from build123d import *

# Parameters (mm, degrees)
F1_DEPTH = 5
F2_R     = 0.7
F3_R     = 2
F4_SIZE  = 0.4
F5_R     = 1.5
F6_DEPTH = 2.001


with BuildPart() as f1:
    # F0 (on Top) → F1 (new body)
    with BuildSketch(Plane.XY):
        with BuildLine():
            ThreePointArc((-7.5, -8), (-3.665936, -1.814164), (-5.040446, 5.332537))
            Line((-5.040446, 5.332537), (-6.5, 3.872983))
            ThreePointArc((-6.5, 3.872983), (-13.5, -8), (-20.5, 3.872983))
            Line((-20.5, 3.872983), (-21.959554, 5.332537))
            ThreePointArc((-21.959554, 5.332537), (-22.255723, -4.830871), (-13.5, -10))
            ThreePointArc((-13.5, -10), (-10.337722, -9.486833), (-7.5, -8))
        make_face()
        with BuildLine():
            Line((7.5, -8), (-7.5, -8))
            ThreePointArc((-7.5, -8), (-10.337722, -9.486833), (-13.5, -10))
            Line((-13.5, -10), (13.5, -10))
            ThreePointArc((13.5, -10), (10.337722, -9.486833), (7.5, -8))
        make_face()
        with BuildLine():
            ThreePointArc((5.040446, 5.332537), (3.665936, -1.814164), (7.5, -8))
            ThreePointArc((7.5, -8), (10.337722, -9.486833), (13.5, -10))
            ThreePointArc((13.5, -10), (22.255723, -4.830871), (21.959554, 5.332537))
            Line((21.959554, 5.332537), (20.5, 3.872983))
            ThreePointArc((20.5, 3.872983), (13.5, -8), (6.5, 3.872983))
            Line((6.5, 3.872983), (5.040446, 5.332537))
        make_face()
    extrude(amount=F1_DEPTH)

    # F2
    f2_edges = [f1.edges().sort_by_distance(p)[0] for p in [
        (5.040446, 5.332537, 2.5),
        (6.5, 3.872983, 2.5),
        (20.5, 3.872983, 2.5),
        (21.959554, 5.332537, 2.5),
        (-5.040446, 5.332537, 2.5),
        (-6.5, 3.872983, 2.5),
        (-21.959554, 5.332537, 2.5),
        (-20.5, 3.872983, 2.5),
    ]]
    fillet(f2_edges, radius=F2_R)

    # F3
    f3_edges = [f1.edges().sort_by_distance(p)[0] for p in [
        (-7.5, -8, 2.5),
        (7.5, -8, 2.5),
    ]]
    fillet(f3_edges, radius=F3_R)

    # F4
    f4_edges = [f1.edges().sort_by_distance(p)[0] for p in [
        (3.504001, -0.282849, 0),
        (4.839746, -7, 0),
        (5.084945, 4.878277, 0),
        (0, -8, 0),
        (5.915081, 4.457902, 0),
        (-4.839746, -7, 0),
        (6.334145, 3.857567, 0),
        (-3.504001, -0.282849, 0),
        (13.5, -8, 0),
        (-5.084945, 4.878277, 0),
        (20.665855, 3.857567, 0),
        (-5.915081, 4.457902, 0),
        (21.084919, 4.457902, 0),
        (-6.334145, 3.857567, 0),
        (21.915055, 4.878277, 0),
        (-13.5, -8, 0),
        (22.015365, -5.242954, 0),
        (-20.665855, 3.857567, 0),
        (0, -10, 0),
        (-21.084919, 4.457902, 0),
        (-22.015365, -5.242954, 0),
        (-21.915055, 4.878277, 0),
        (3.504001, -0.282849, 5),
        (4.839746, -7, 5),
        (5.084945, 4.878277, 5),
        (0, -8, 5),
        (5.915081, 4.457902, 5),
        (-4.839746, -7, 5),
        (6.334145, 3.857567, 5),
        (-3.504001, -0.282849, 5),
        (13.5, -8, 5),
        (-5.084945, 4.878277, 5),
        (20.665855, 3.857567, 5),
        (-5.915081, 4.457902, 5),
        (21.084919, 4.457902, 5),
        (-6.334145, 3.857567, 5),
        (21.915055, 4.878277, 5),
        (-13.5, -8, 5),
        (22.015365, -5.242954, 5),
        (-20.665855, 3.857567, 5),
        (0, -10, 5),
        (-21.084919, 4.457902, 5),
        (-22.015365, -5.242954, 5),
        (-21.915055, 4.878277, 5),
    ]]
    chamfer(f4_edges, length=F4_SIZE)

    # F5 (on face) → F6 (cut, through all)
    with BuildSketch(Plane(origin=(0, -8, 0), x_dir=(-1, 0, 0), z_dir=(0, 1, 0))):
        with Locations((0, 2.5)):
            Circle(F5_R)
    extrude(amount=-F6_DEPTH, mode=Mode.SUBTRACT)


solid = f1.part
Verification items for the finished model (mm, model axes). A direction names the side the tool comes from. Give positions to 0.01 mm unless a question says otherwise; leave off trailing zeros. Write each loop counter-clockwise with the first axis right and the second up, starting at its lowest first coordinate (ties: lowest second). Pieces come first, ordered by that corner, then holes.
(1) Material ranges on line 1 (X direction, y = 0, z = 2.75); line 2 (X direction, y = 1.75, z = 0.75); line 3 (Y direction, x = 13.5, z = 2.95), recorded low to high.
(2) Cross-section at A-A (y = 0). State how many separate pieces and enclosed holes the cut face has, plus the area to 3 significant figures.
(3) Access from +Z, -Z, +X, -X, +Y, -Y to the whole of each face (thin tool, end or side, straight path). Record for faces 1 (the face through (3.5, -0.2, 2.5)), 2 (the face through (2, -9, 0)), 3 (the face through (1, -8, 1)).
(4) Cross-section at B-B (z = 2.5). Enter the section's corners in (x, y).
(5) Mould release check, pull along X, two halves, no side actions. Record for faces 4 (the face through (21.94, -5.36, 2.47)), 5 (the face through (21.924, 4.877, 2.529)), 6 (the face through (5.09, 4.88, 2.53)), 7 (the face through (-0.2, -10, 0.6)): +X half, -X half, draft (parallel to the pull), parting line (faces both ways), or undercut.
(6) Gauge pin test, flat end, axial feed: pin 1 (1 mm diameter, centred on x = 13.5, z = 4, fed in from +Y). Record the tip position at first contact, or that the pin passes through.
Worked out:
1. line 1: x = -23.5 to -21.5, -5.5 to -3.5, 3.5 to 5.5, 21.5 to 23.5
1. line 2: x = -23.35 to -21.31, -5.69 to -3.65, 3.65 to 5.69, 21.31 to 23.35
1. line 3: y = -10 to -8
2. separate pieces: 4
2. enclosed holes: 0
2. area: 38.7 mm2
3. face 1: +Z, -Z
3. face 2: -Z, +X, -X, +Y, -Y
3. face 3: +Z, -Z, +Y
4. outline: (-22.43, 4.5) arc R10 ccw to (-13.5, -10) - (-1.5, -10) - (-1.5, -8) - (-3.11, -8) arc R2 cw to (-4.84, -5) arc R10 ccw to (-4.57, 4.5) arc R0.7 ccw to (-5.69, 4.68) - (-6.14, 4.23) arc R0.7 ccw to (-6.28, 3.44) arc R8 cw (long way) to (-20.72, 3.44) arc R0.7 ccw to (-20.86, 4.23) - (-21.31, 4.68) arc R0.7 ccw to start; (1.5, -10) - (13.5, -10) arc R10 ccw to (22.43, 4.5) arc R0.7 ccw to (21.31, 4.68) - (20.86, 4.23) arc R0.7 ccw to (20.72, 3.44) arc R8 cw (long way) to (6.28, 3.44) arc R0.7 ccw to (6.14, 4.23) - (5.69, 4.68) arc R0.7 ccw to (4.57, 4.5) arc R10 ccw to (4.84, -5) arc R2 cw to (3.11, -8) - (1.5, -8) - close
5. face 4: +X half
5. face 5: undercut
5. face 6: undercut
5. face 7: draft
6. pin 1: stops at y = -7.98
